Autodesk Inventor part; units mm, degrees
ref_plane "YZ Plane" through (0, 0, 0) normal (1, 0, 0) x (0, 1, 0)
ref_plane "XZ Plane" through (0, 0, 0) normal (0, 1, 0) x (-1, 0, 0)
ref_plane "XY Plane" through (0, 0, 0) normal (0, 0, 1) x (1, 0, 0)
sketch "Sketch1" plane through (0, 0, 0) normal (0, 0, 1) x (1, 0, 0)
  line L0 (0, 0) -> (23.54, 0)
  line L1 (23.54, 0) -> (23.54, 14.75)
  line L2 (23.54, 14.75) -> (0, 14.75)
  line L3 (0, 14.75) -> (0, 0)
  dimension "d0" = 23.54
  dimension "d1" = 14.75
extrude "Extrusion1" add sketch "Sketch1" against normal blind 14.65
sketch "Sketch2" plane through (0, 14.75, 0) normal (0, 1, 0) x (1, 0, 0)
  line L0 (23.54, 0) -> (0, 0)
  line L1 (0, 0) -> (0, 14.65)
  line L2 (23.54, 14.65) -> (0, 14.65)
  line L3 (0, 0) -> (5.8865, 0)
  line L4 (5.8865, 0) -> (5.8865, 14.65)
  line L5 (5.8865, 14.65) -> (0, 14.65)
  line L6 (0, 14.65) -> (0, 0)
  line L7 (23.54, 14.65) -> (17.6472, 14.65)
  line L8 (17.6472, 14.65) -> (17.6472, 0)
  line L9 (17.6472, 0) -> (23.54, 0)
  line L10 (23.54, 0) -> (23.54, 14.65)
  line L11 (5.8865, 0) -> (17.6472, 0)
  line L12 (17.6472, 0) -> (17.6472, 7.325)
  line L13 (17.6472, 7.325) -> (5.8865, 7.325)
  line L14 (5.8865, 7.325) -> (5.8865, 0)
  dimension "d4" = 5.8864
  dimension "d5" = 5.8928
extrude "Extrusion2" cut sketch "Sketch2" against normal blind 9.57 contours L0 L8 L2 L10 | L0 L4 L13 L8 | L0 L1 L2 L4
properties part number "BOB-10031 USB Micro B Breakout"
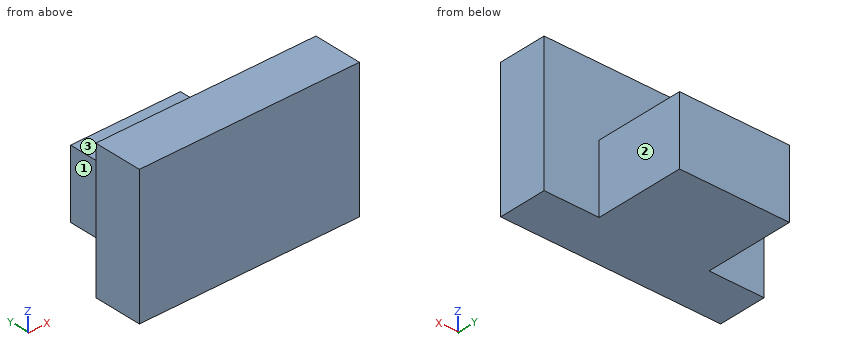
Model file for the job. Use its own axes, mm. Face numbers are marked on the shaded views. A direction names the side the tool comes from. Give positions to 0.01 mm unless a question says otherwise; leave off trailing zeros. Loops run counter-clockwise (first coordinate to the right, second up) from the corner with the lowest first, then second, coordinate; pieces in that order, holes last.
1) Flat gauge pins, fed straight in: pin 1 Ø1.5 at (y, z) = (10.5, -11.5) entering from -X; pin 2 Ø3 at (y, z) = (5, -7.5) entering from -X; pin 3 Ø3.5 at (y, z) = (11.5, -11) entering from +X; pin 4 Ø3 at (x, y) = (9, 9) entering from +Z (3 decimals). Where does each tip first touch, or does it go through?
2) Saw through at D-D (z = -1). Write the cut outline in (x, y).
3) Saw through at A-A (x = 15.5). Write the cut outline in (y, z) (3 decimals).
4) Tool access for the marked faces 1, 2 and 3: list every direction of +Z, -Z, +X, -X, +Y, -Y with a clear straight run to the whole face (end or side of a thin tool).
5) Wall check: line 1 (Y direction, x = 4.25, z = -4.25); line 2 (Z direction, x = 16.25, y = 8.75) (3 decimals); line 3 (X direction, y = 12, z = -11.75). Give the ranges that are in metal, low to high.
6) Saw through at B-B (z = -12.5). Write the cut outline in (x, y).
Answer block:
1. pin 1: stops at x = 5.89
1. pin 2: stops at x = 0
1. pin 3: stops at x = 17.65
1. pin 4: stops at z = -7.325
2. outline: (0, 0) - (23.54, 0) - (23.54, 5.18) - (0, 5.18) - close
3. outline: (0, -14.65) - (14.75, -14.65) - (14.75, -7.325) - (5.18, -7.325) - (5.18, 0) - (0, 0) - close
4. face 1: +Z, -Z, -X, +Y
4. face 2: +Z, -Z, +X, +Y
4. face 3: +Z, +X, -X, +Y
5. line 1: y = 0 to 5.18
5. line 2: z = -14.65 to -7.325
5. line 3: x = 5.89 to 17.65
6. outline: (0, 0) - (23.54, 0) - (23.54, 5.18) - (17.65, 5.18) - (17.65, 14.75) - (5.89, 14.75) - (5.89, 5.18) - (0, 5.18) - close
